```python
from build123d import *

# Parameters (mm, degrees)
ESQUISSE1_R             = 10
BOSS_EXTRU_1_DEPTH      = 10
D_ME1_FACE_RADIUS       = 10
D_ME1_HEIGHT            = 10
ESQUISSE2_R             = 2.52
ENL_V_MAT_EXTRU_1_DEPTH = 10


with BuildPart() as part:
    # Esquisse1 → Boss.-Extru.1 (new body)
    with BuildSketch(Plane.XY):
        Circle(ESQUISSE1_R)
    extrude(amount=BOSS_EXTRU_1_DEPTH)

    # Dôme1: a dome of height H over a round flat face of radius A is a cap of a sphere of radius (A * A + H * H) / (2 * H)
    d_me1_r = (D_ME1_FACE_RADIUS * D_ME1_FACE_RADIUS + D_ME1_HEIGHT * D_ME1_HEIGHT) / (2 * D_ME1_HEIGHT)
    d_me1_base = Plane((0, 0, 10), z_dir=(0, 0, 1))
    with Locations(d_me1_base.offset(D_ME1_HEIGHT - d_me1_r)):
        d_me1_ball = Sphere(d_me1_r, mode=Mode.PRIVATE)
    add(split(d_me1_ball, bisect_by=d_me1_base, keep=Keep.TOP, mode=Mode.PRIVATE))

    # Esquisse2 → Enlèv. mat.-Extru.1 (cut)
    with BuildSketch(Plane(origin=(0, 0, 0), x_dir=(-1, 0, 0), z_dir=(0, 0, -1))):
        Circle(ESQUISSE2_R)
    extrude(amount=-ENL_V_MAT_EXTRU_1_DEPTH, mode=Mode.SUBTRACT)


solid = part.part
```
Here's how the part is built. I have some questions about the finished solid (model axes, mm). Coordinates: 2 decimals unless noted, no trailing zeros. Loops run counter-clockwise (first coordinate to the right, second up) from the corner with the lowest first, then second, coordinate; pieces in that order, holes last. Notation, with made-up numbers: (-5, -14.5) - (32, -14.5) arc R23 ccw to (32, -0.5) - close; hole circle Ø8 at (-31.5, -20.5). An arc over 180 degrees is marked (long way). Return JSON: item names as keys, results as strings. Group by question number.
Item 1: Will these pins go through, and if not, where does the flat tip stop? P1, Ø1.5, axis at x = -0.5, y = 0.5, coming from the -Z side; P2, Ø5, axis at y = 4.5, z = 7.5, coming from the -X side; P3, Ø4, axis at y = -6.5, z = 11.5, coming from the -X side.
Item 2: If we section it at B-B on y = 1.75: Write out the boundary of the cut face in (x, z).
Item 3: I need wall thicknesses on line 1 (Y direction, x = 0, z = 7.25); line 2 (X direction, y = 2.25, z = 8.5); line 3 (Y direction, x = 1, z = 8.25). Which ranges of each line are inside material? Lowest first, please. Write a range as from..to.
Item 4: If we section it at D-D on y = -4: Write out the boundary of the cut face in (x, z).
Item 5: If we section it at A-A on x = 0: Write out the boundary of the cut face in (y, z), and give its area (3 significant figures).
Item 6: We'd pull the mould along Y, two halves only. Please class faces 1 (the face through (2, -2, 0)), 2 (the face through (-2.17, -9.76, 4.93)), 3 (the face through (0, 0, 10)): +Y half, -Y half, draft (parallel to the pull), parting line (faces both ways), or undercut.
Item 7: If we section it at C-C on x = 8: Write out the boundary of the cut face in (y, z).
Calculated:
{
 "1": {"P1": "stops at z = 10", "P2": "stops at x = -9.8", "P3": "stops at x = -8.84"},
 "2": {"outline": "(-9.85, 0) - (-1.81, 0) - (-1.81, 10) - (1.81, 10) - (1.81, 0) - (9.85, 0) - (9.85, 10) arc R9.85 ccw to (-9.85, 10) - close"},
 "3": {"line 1": "y = -10..-2.52, 2.52..10", "line 2": "x = -9.74..-1.13, 1.13..9.74", "line 3": "y = -9.95..-2.31, 2.31..9.95"},
 "4": {"outline": "(-9.17, 0) - (9.17, 0) - (9.17, 10) arc R9.17 ccw to (-9.17, 10) - close"},
 "5": {"outline": "(-10, 0) - (-2.52, 0) - (-2.52, 10) - (2.52, 10) - (2.52, 0) - (10, 0) - (10, 10) arc R10 ccw to (-10, 10) - close", "area": "307 mm^2"},
 "6": {"face 1": "draft", "face 2": "parting line", "face 3": "undercut"},
 "7": {"outline": "(-6, 0) - (6, 0) - (6, 10) arc R6 ccw to (-6, 10) - close"}
}
